from build123d import *

# Parameters (mm, degrees)
F1_DEPTH = 10.16
F2_DEPTH = 35.56
F3_DEPTH = 15.24
F4_DEPTH = 25.4


with BuildPart() as f1:
    # F0 (on Top) → F1 (new body)
    with BuildSketch(Plane.XY):
        with BuildLine():
            Line((-91.44, -20.32), (-91.44, 0))
            Line((-91.44, 0), (-116.84, 0))
            Line((-116.84, 0), (-116.84, -12.7))
            Line((-116.84, -12.7), (-106.68, -12.7))
            ThreePointArc((-106.68, -12.7), (-101.2918463274, -14.9318463274), (-99.06, -20.32))
            ThreePointArc((-99.06, -20.32), (-101.2918463274, -25.7081536726), (-106.68, -27.94))
            Line((-106.68, -27.94), (-116.84, -27.94))
            Line((-116.84, -27.94), (-116.84, -40.64))
            Line((-116.84, -40.64), (-91.44, -40.64))
            Line((-91.44, -40.64), (-91.44, -20.32))
        make_face()
    extrude(amount=F1_DEPTH)



with BuildPart() as f1b:
    # F0 (on Top) → F1, piece 2 (new body)
    with BuildSketch(Plane.XY):
        with BuildLine():
            Line((0, -12.7), (0, 0))
            Line((0, 0), (-25.4, 0))
            Line((-25.4, 0), (-25.4, -20.32))
            Line((-25.4, -20.32), (-25.4, -40.64))
            Line((-25.4, -40.64), (0, -40.64))
            Line((0, -40.64), (0, -27.94))
            Line((0, -27.94), (-10.16, -27.94))
            ThreePointArc((-10.16, -27.94), (-15.5481536726, -25.7081536726), (-17.78, -20.32))
            ThreePointArc((-17.78, -20.32), (-15.5481536726, -14.9318463274), (-10.16, -12.7))
            Line((-10.16, -12.7), (0, -12.7))
        make_face()
    extrude(amount=F1_DEPTH)


with BuildPart() as f1_1:
    add(f1.part)

    add(f1b.part)  # F2 merges F1b
    # F0 (on Top) → F2 (join)
    with BuildSketch(Plane.XY):
        Polygon((-25.4, -20.32), (-25.4, 0), (-58.42, 0), (-91.44, 0), (-91.44, -20.32), (-91.44, -40.64), (-58.42, -40.64), (-25.4, -40.64), align=None)
        Polygon((-33.02, -7.62), (-33.02, -20.32), (-33.02, -33.02), (-58.42, -33.02), (-83.82, -33.02), (-83.82, -20.32), (-83.82, -7.62), (-58.42, -7.62), align=None, mode=Mode.SUBTRACT)
    extrude(amount=F2_DEPTH)

    # F0 (on Top) → F3 (join)
    with BuildSketch(Plane.XY):
        with BuildLine():
            Line((-58.42, -9.652), (-58.42, -7.62))
            Line((-58.42, -7.62), (-83.82, -7.62))
            Line((-83.82, -7.62), (-83.82, -20.32))
            Line((-83.82, -20.32), (-83.82, -33.02))
            Line((-83.82, -33.02), (-58.42, -33.02))
            Line((-58.42, -33.02), (-58.42, -30.988))
            ThreePointArc((-58.42, -30.988), (-69.088, -20.32), (-58.42, -9.652))
        make_face()
        with BuildLine():
            Line((-33.02, -33.02), (-33.02, -20.32))
            Line((-33.02, -20.32), (-33.02, -7.62))
            Line((-33.02, -7.62), (-58.42, -7.62))
            Line((-58.42, -7.62), (-58.42, -9.652))
            ThreePointArc((-58.42, -9.652), (-50.8765848583, -12.7765848583), (-47.752, -20.32))
            ThreePointArc((-47.752, -20.32), (-50.8765848583, -27.8634151417), (-58.42, -30.988))
            Line((-58.42, -30.988), (-58.42, -33.02))
            Line((-58.42, -33.02), (-33.02, -33.02))
        make_face()
    extrude(amount=F3_DEPTH)

    # F0 (on Top) → F4 (join)
    with BuildSketch(Plane.XY):
        with BuildLine():
            Line((-58.42, -15.24), (-58.42, -9.652))
            ThreePointArc((-58.42, -9.652), (-69.088, -20.32), (-58.42, -30.988))
            Line((-58.42, -30.988), (-58.42, -25.4))
            ThreePointArc((-58.42, -25.4), (-63.5, -20.32), (-58.42, -15.24))
        make_face()
        with BuildLine():
            ThreePointArc((-47.752, -20.32), (-50.8765848583, -12.7765848583), (-58.42, -9.652))
            Line((-58.42, -9.652), (-58.42, -15.24))
            ThreePointArc((-58.42, -15.24), (-54.8278975516, -16.7278975516), (-53.34, -20.32))
            ThreePointArc((-53.34, -20.32), (-54.8278975516, -23.9121024484), (-58.42, -25.4))
            Line((-58.42, -25.4), (-58.42, -30.988))
            ThreePointArc((-58.42, -30.988), (-50.8765848583, -27.8634151417), (-47.752, -20.32))
        make_face()
    extrude(amount=F4_DEPTH)


solid = f1_1.part
Geometry check sheet. Reference: the model listing, model coordinates, mm. A direction names the side the tool comes from. Coordinates: 2 decimals unless noted, no trailing zeros. Order: outer loops, then holes, each group sorted by start corner. A loop starts at its lowest first (then second) coordinate and runs counter-clockwise, first axis right, second up. Notation, with made-up numbers: M 59,-13 L 76,-13 A11 ccw 76,4 Z; hole C 3.5,-36.75 d3. An arc over 180 degrees is marked long. Use CSV: the item, a comma, the result in double quotes.
Item 1: Thickness scan on line 1 along X through (y, z) = (-12.5, 30); line 2 along Y through (x, z) = (-42, 22.5); line 3 along X through (y, z) = (-7.5, 19). Record the ranges inside material, lowest first.
Returned:
line 1,"x = -91.44 to -83.82, -33.02 to -25.4"
line 2,"y = -40.64 to -33.02, -7.62 to 0"
line 3,"x = -91.44 to -25.4"
Item 2: Cross-section at A-A on z = 21. Record the cut outline in (x, y).
Returned:
outline,"M -91.44,-40.64 L -25.4,-40.64 L -25.4,0 L -91.44,0 Z; C -58.42,-20.32 d21.34; hole M -83.82,-33.02 L -33.02,-33.02 L -33.02,-7.62 L -83.82,-7.62 Z; hole C -58.42,-20.32 d10.16"
Item 3: Gauge pin test, flat ends, axial feed: pin 1 Ø7.5 at (y, z) = (-25.5, 23.5) entering from +X; pin 2 Ø7.5 at (x, y) = (-105, -24.5) entering from +Z; pin 3 Ø16.5 at (y, z) = (-22.5, 30.5) entering from -X. Record the tip position at first contact, or that the pin passes through.
Returned:
pin 1,"stops at x = -25.4"
pin 2,"stops at z = 10.16"
pin 3,"stops at x = -91.44"
Item 4: Cross-section at D-D on y = -18. Record the cut outline in (x, z), then the cut area to 3 significant figures.
Returned:
outline,"M -99.42,0 L -62.94,0 L -62.94,25.4 L -68.83,25.4 L -68.83,15.24 L -83.82,15.24 L -83.82,35.56 L -91.44,35.56 L -91.44,10.16 L -99.42,10.16 Z; M -53.9,0 L -17.42,0 L -17.42,10.16 L -25.4,10.16 L -25.4,35.56 L -33.02,35.56 L -33.02,15.24 L -48.01,15.24 L -48.01,25.4 L -53.9,25.4 Z"
area,"1,460 mm2"
Item 5: Tool access check on faces 1 (the flat face through (-5, -27.94, 5)), 2 (the flat face through (-25.4, -21, 23)), 3 (the flat face through (-98.7, -20, 10.16)). Record the directions out of +Z, -Z, +X, -X, +Y, -Y that give a thin tool (end or side, any length) a straight path to the whole face; none if there is none.
Returned:
face 1,"+Z, -Z, +X"
face 2,"+Z, +X, +Y, -Y"
face 3,"+Z, -X, +Y, -Y"
Item 6: Mould release check, pull along X, two halves, no side actions. Record for faces 4 (the flat face through (0, -34, 5)), 5 (the flat face through (-59, -29, 0)), 6 (the flat face through (-116.84, -34, 5)), 7 (the flat face through (-56, -25, 25.4)): pulls with the +X half, pulls with the -X half, needs draft (parallel to the pull), parting line crosses it, or undercut.
Returned:
face 4,"pulls with the +X half"
face 5,"needs draft"
face 6,"pulls with the -X half"
face 7,"undercut"
Item 7: Cross-section at C-C on z = 29.5. Record the cut outline in (x, y), then the cut area to 3 significant figures.
Returned:
outline,"M -91.44,-40.64 L -25.4,-40.64 L -25.4,0 L -91.44,0 Z; hole M -83.82,-33.02 L -33.02,-33.02 L -33.02,-7.62 L -83.82,-7.62 Z"
area,"1,390 mm2"
Item 8: Cross-section at B-B on x = -101. Record the cut outline in (y, z).
Returned:
outline,"M -40.64,0 L -25.4,0 L -25.4,10.16 L -40.64,10.16 Z; M -15.24,0 L 0,0 L 0,10.16 L -15.24,10.16 Z"
